Can you work these out from the model? Positions are in its coordinate system, mm. Coordinates: 2 decimals unless noted, no trailing zeros. Order: outer loops, then holes, each group sorted by start corner. A loop starts at its lowest first (then second) coordinate and runs counter-clockwise, first axis right, second up. Notation, with made-up numbers: (-14, 10.25) -> (45, 10.25) arc R12 cw to (45, 23.25) -> close; hole circle Ø10 at (57.25, -14.5). An arc over 180 degrees is marked (long way). Return JSON: item names as keys, results as strings. Group by question number.
1) If we section it at B-B, the plane x = 4: Please give me the cut outline in (y, z).
2) If we section it at A-A, the plane z = -1.27: Please give me the cut outline in (x, y), then the cut area to 3 significant figures.
3) For pin 1 (1 mm diameter, centred on x = 11.12, z = -1.27, fed in from +Y), with a flat end and sliding along its axis, tell me the tip position at first contact or that it passes through.
4) If we section it at D-D, the plane x = 5.75: Please give me the cut outline in (y, z), then the cut area to 3 significant figures.
5) If I drill on probe 1 along X at (y, z) = (-0.6, -1.27); probe 2 along Z at (x, y) = (3.5, -1.05); probe 3 along Z at (x, y) = (3, -2.1), over which ranges is the centre line in solid material (lowest first)? Write a range as from..to.
6) If we section it at C-C, the plane z = -4.1: Please give me the cut outline in (x, y), then the cut area to 3 significant figures.
7) Thinking about a two-plate mould opening in X: for faces 1 (the flat face through (12.394, -1, -3)), 2 (the flat face through (11, -1, -5.08)), 3 (the cylindrical face through (8.825, -1.417, -4.574)), which applies, +X half, -X half, draft (parallel to the pull), parting line (faces both ways), or undercut?
from build123d import *

# Parameters (mm, degrees)
EXTRUDE1_DEPTH       = 2.794
HOLE1_D              = 1.60274
EXTRUDE2_DEPTH       = 2.794
LPATTERN1_COUNT      = 5
LPATTERN1_PITCH      = 2.54
LPATTERN1_COUNT_DIR2 = 2
LPATTERN1_PITCH_DIR2 = 2.54
LPATTERN2_COUNT      = 35
LPATTERN2_PITCH      = 2.54


with BuildPart() as part:
    # Sketch1 → Extrude1 (new body)
    with BuildSketch(Plane(origin=(0, 0, 0), x_dir=(1, 0, 0), z_dir=(0, 1, 0))):
        Polygon((12.394373708, 0.40005), (12.234353708, 0.40005), (12.088747416, 0), (0, 0), (-0.145606292, 0.40005), (-0.305626292, 0.40005), (-0.305626292, 4.67995), (-0.145606292, 4.67995), (0, 5.08), (12.088747416, 5.08), (12.234353708, 4.67995), (12.394373708, 4.67995), align=None)
    extrude(amount=-EXTRUDE1_DEPTH)

    # Hole1 (through all)
    with Locations(Plane(origin=(0.964373708, 0, -1.27), x_dir=(0, 0, 1), z_dir=(0, 1, 0))):
        with Locations((0, 0)):
            hole1 = Hole(HOLE1_D / 2)

    # Sketch4 → Extrude2 (cut)
    with BuildSketch(Plane(origin=(0, 0, 0), x_dir=(1, 0, 0), z_dir=(0, 1, 0))):
        Polygon((1.928772816, 0), (2.5399746, 0), (2.394368308, 0.40005), (2.074379108, 0.40005), align=None)
        Polygon((2.074379108, 4.67995), (2.394368308, 4.67995), (2.5399746, 5.08), (1.928772816, 5.08), align=None)
    extrude2 = extrude(amount=-EXTRUDE2_DEPTH, mode=Mode.SUBTRACT)

    # LPattern1: Hole1 5 × 2
    with Locations(*[(i * LPATTERN1_PITCH, 0, -j * LPATTERN1_PITCH_DIR2) for i in range(LPATTERN1_COUNT) for j in range(LPATTERN1_COUNT_DIR2) if (i, j) != (0, 0)]):
        add(hole1, mode=Mode.SUBTRACT)

    # LPattern2: Extrude2 ×35
    with Locations(*[(i * LPATTERN2_PITCH, 0, 0) for i in range(1, LPATTERN2_COUNT)]):
        add(extrude2, mode=Mode.SUBTRACT)


solid = part.part
Result sheet:
{
 "1": {"outline": "(-2.79, -5.08) -> (0, -5.08) -> (0, -4.44) -> (-2.79, -4.44) -> close; (-2.79, -3.18) -> (0, -3.18) -> (0, -1.9) -> (-2.79, -1.9) -> close; (-2.79, -0.64) -> (0, -0.64) -> (0, 0) -> (-2.79, 0) -> close"},
 "2": {"outline": "(-0.31, -2.79) -> (0.16, -2.79) -> (0.16, 0) -> (-0.31, 0) -> close; (1.77, -2.79) -> (2.7, -2.79) -> (2.7, 0) -> (1.77, 0) -> close; (4.31, -2.79) -> (5.24, -2.79) -> (5.24, 0) -> (4.31, 0) -> close; (6.85, -2.79) -> (7.78, -2.79) -> (7.78, 0) -> (6.85, 0) -> close; (9.39, -2.79) -> (10.32, -2.79) -> (10.32, 0) -> (9.39, 0) -> close; (11.93, -2.79) -> (12.39, -2.79) -> (12.39, 0) -> (11.93, 0) -> close", "area": "13.1 mm2"},
 "3": {"pin 1": "passes through"},
 "4": {"outline": "(-2.79, -5.08) -> (0, -5.08) -> (0, -4.56) -> (-2.79, -4.56) -> close; (-2.79, -3.06) -> (0, -3.06) -> (0, -2.02) -> (-2.79, -2.02) -> close; (-2.79, -0.52) -> (0, -0.52) -> (0, 0) -> (-2.79, 0) -> close", "area": "5.86 mm2"},
 "5": {"probe 1": "x = -0.31..0.16, 1.77..2.7, 4.31..5.24, 6.85..7.78, 9.39..10.32, 11.93..12.39", "probe 2": "z = -5.08..-4.61, -3.01..-2.07, -0.47..0", "probe 3": "z = -5.08..-4.43, -3.19..-1.89, -0.65..0"},
 "6": {"outline": "(-0.31, -2.79) -> (0.22, -2.79) -> (0.22, 0) -> (-0.31, 0) -> close; (1.71, -2.79) -> (2.76, -2.79) -> (2.76, 0) -> (1.71, 0) -> close; (4.25, -2.79) -> (5.3, -2.79) -> (5.3, 0) -> (4.25, 0) -> close; (6.79, -2.79) -> (7.84, -2.79) -> (7.84, 0) -> (6.79, 0) -> close; (9.33, -2.79) -> (10.38, -2.79) -> (10.38, 0) -> (9.33, 0) -> close; (11.87, -2.79) -> (12.39, -2.79) -> (12.39, 0) -> (11.87, 0) -> close", "area": "14.6 mm2"},
 "7": {"face 1": "+X half", "face 2": "draft", "face 3": "undercut"}
}
